```python
from build123d import *

# Parameters (mm, degrees)
SKETCH_1_W      = 5
SKETCH_1_H      = 12.4
SKETCH_1_R      = 1.2
EXTRUDE_1_DEPTH = 4
SKETCH_2_R      = 4
SKETCH_2_R_2    = 1.2
EXTRUDE_2_DEPTH = 3
FILLET_1_R      = 5


with BuildPart() as part:
    # Эскиз1 → Бобышка-Вытянуть1 (new body)
    with BuildSketch(Plane(origin=(0, 0, 0), x_dir=(1, 0, 0), z_dir=(0, 1, 0))):
        Polygon((-11.2, 6.2), (-6.2, 6.2), (0, 6.2), (16.4, 6.2), (21.4, 6.2), (21.4, -6.2), (16.4, -6.2), (6e-09, -6.2), (-6.2, -6.2), (-11.2, -6.2), (-11.2, -9.2), (24, -9.2), (24, 9.2), (-11.2, 9.2), align=None)
        Polygon((-6.2, 0), (-6.2, 6.2), (-11.2, 6.2), (-11.2, -6.2), (-6.2, -6.2), align=None)
        with Locations((18.9, 0)):
            Rectangle(SKETCH_1_W, SKETCH_1_H)
        with Locations((20, 0)):
            Circle(SKETCH_1_R, mode=Mode.SUBTRACT)
        with BuildLine():
            Line((16.4, 6.2), (0, 6.2))
            ThreePointArc((0, 6.2), (2.230840311, 5.784751637), (4.162857143, 4.594629518))
            Line((4.162857143, 4.594629518), (8.007142857, 1.111603916))
            ThreePointArc((8.007142857, 1.111603916), (8.37126115, 0.607982613), (8.5, 0))
            ThreePointArc((8.5, 0), (8.37126115, -0.607982613), (8.007142857, -1.111603916))
            Line((8.007142857, -1.111603916), (4.162857143, -4.594629518))
            ThreePointArc((4.162857143, -4.594629518), (2.230840314, -5.784751636), (6e-09, -6.2))
            Line((6e-09, -6.2), (16.4, -6.2))
            Line((16.4, -6.2), (16.4, 6.2))
        make_face()
        with BuildLine():
            Line((0, 6.2), (-6.2, 6.2))
            Line((-6.2, 6.2), (-6.2, 0))
            ThreePointArc((-6.2, 0), (-4.384062043, 4.384062043), (0, 6.2))
        make_face()
        with BuildLine():
            ThreePointArc((6e-09, -6.2), (-4.384062041, -4.384062046), (-6.2, 0))
            Line((-6.2, 0), (-6.2, -6.2))
            Line((-6.2, -6.2), (6e-09, -6.2))
        make_face()
    extrude(amount=EXTRUDE_1_DEPTH)

    # Эскиз2 → Бобышка-Вытянуть2 (add)
    with BuildSketch(Plane(origin=(0, 4, 0), x_dir=(1, 0, 0), z_dir=(0, 1, 0))):
        with Locations((20, 0)):
            Circle(SKETCH_2_R)
        with Locations((20, 0)):
            Circle(SKETCH_2_R_2, mode=Mode.SUBTRACT)
    extrude(amount=EXTRUDE_2_DEPTH)

    # Скругление1
    fillet_1_edges = [part.edges().sort_by_distance(p)[0] for p in [
        (24, 2, 9.2),
        (-11.2, 2, 9.2),
        (-11.2, 2, -9.2),
        (24, 2, -9.2),
    ]]
    fillet(fillet_1_edges, radius=FILLET_1_R)


solid = part.part
```
Check sheet for the modelled part. Datum: model origin and axes. Units: mm. A direction names the side the tool comes from. Give positions to 0.01 mm unless a question says otherwise; leave off trailing zeros. Write each loop counter-clockwise with the first axis right and the second up, starting at its lowest first coordinate (ties: lowest second). Pieces come first, ordered by that corner, then holes. Notation, with made-up numbers: (57.5, 37.25) -> (66.5, 37.25) arc R29 cw to (66.5, 58.25) -> close; hole circle Ø6 at (22.25, -33.75). An arc over 180 degrees is marked (long way). Use CSV: the item, a comma, the result in double quotes. Start each with the question number.
Q1. Cross-section at B-B on z = 5.75. Enter the section's corners in (x, y).
Q2. Cross-section at D-D on x = 19.5. Enter the section's corners in (y, z), and give its area (3 significant figures).
Q3. Tool access check on faces 5 (the cylindrical face through (16.8, 5.5, 2.4)), 6 (the flat face through (7, 2, -9.2)). Record the directions out of +Z, -Z, +X, -X, +Y, -Y that give a thin tool (end or side, any length) a straight path to the whole face; none if there is none.
Q4. Cross-section at C-C on x = 2. Enter the section's corners in (y, z), and give its area (3 significant figures).
Q5. Depth check by flat-ended pin: P1, Ø3, axis at x = 20, z = 0, coming from the -Y side; P2, Ø1, axis at x = 16, y = 5, coming from the -Z side; P3, Ø5.5, axis at x = 10.5, z = -2.5, coming from the +Y side. Enter the tip coordinate at first touch or a pass-through.
Q6. Cross-section at A-A on y = 1.5. Enter the section's corners in (x, z), and give its area (3 significant figures).
Q7. Release check for a two-part mould opening along Z. For faces 1 (the flat face through (6, 2, 9.2)), 2 (the flat face through (6.058, 1.972, -2.877)), 3 (the flat face through (6.11, 1.97, 2.83)), 4 (the flat face through (24, 2, 0)) record: +Z half, -Z half, draft (parallel to the pull), parting line (faces both ways), or undercut.
Q8. Scan lines: line 1 along X through (y, z) = (2.25, 0); line 2 along Z through (x, y) = (20, 4.75); line 3 along X through (y, z) = (2.25, -0.5). Record each from-to range of solid material in increasing order.
Working result:
1,outline,"(-10.95, 0) -> (-2.32, 0) -> (-2.32, 4) -> (-10.95, 4) -> close; (2.32, 0) -> (23.75, 0) -> (23.75, 4) -> (2.32, 4) -> close"
2,outline,"(0, -9.17) -> (4, -9.17) -> (4, -3.97) -> (7, -3.97) -> (7, -1.09) -> (0, -1.09) -> close; (0, 1.09) -> (7, 1.09) -> (7, 3.97) -> (4, 3.97) -> (4, 9.17) -> (0, 9.17) -> close"
2,area,"81.9 mm^2"
3,face 5,"+Y"
3,face 6,"-Z, +X, -X, +Y, -Y"
4,outline,"(0, -9.2) -> (4, -9.2) -> (4, -5.87) -> (0, -5.87) -> close; (0, 5.87) -> (4, 5.87) -> (4, 9.2) -> (0, 9.2) -> close"
4,area,"26.7 mm^2"
5,P1,"stops at y = 0"
5,P2,"stops at z = -1.94"
5,P3,"stops at y = 4"
6,outline,"(-11.2, -4.2) arc R5 ccw to (-6.2, -9.2) -> (19, -9.2) arc R5 ccw to (24, -4.2) -> (24, 4.2) arc R5 ccw to (19, 9.2) -> (-6.2, 9.2) arc R5 ccw to (-11.2, 4.2) -> close; hole (4.16, -4.59) -> (8.01, -1.11) arc R1.5 ccw to (8.01, 1.11) -> (4.16, 4.59) arc R6.2 ccw (long way) to start; hole circle Ø2.4 at (20, 0)"
6,area,"491 mm^2"
7,face 1,"+Z half"
7,face 2,"undercut"
7,face 3,"undercut"
7,face 4,"draft"
8,line 1,"x = -11.2 to -6.2, 8.5 to 18.8, 21.2 to 24"
8,line 2,"z = -4 to -1.2, 1.2 to 4"
8,line 3,"x = -11.2 to -6.18, 8.41 to 18.91, 21.09 to 24"
